Part model, mm, in its own coordinate system. A direction names the side the tool comes from. Give positions to 0.01 mm unless a question says otherwise; leave off trailing zeros. Write each loop counter-clockwise with the first axis right and the second up, starting at its lowest first coordinate (ties: lowest second). Pieces come first, ordered by that corner, then holes. Notation, with made-up numbers: M 16.5,8 L 40.5,8 A24 cw 40.5,33 Z; hole C 76,73.5 d6. An arc over 180 degrees is marked long. Use a Markdown table: item, result.
```python
from build123d import *

# Parameters (mm, degrees)
SKETCH_2_R          = 2.75
CUT_EXTRUDE_1_DEPTH = 10


with BuildPart() as part:
    # 草图1 → 旋转1 (revolve)
    with BuildSketch(Plane.XY, mode=Mode.PRIVATE) as revolve_1_sk:
        Polygon((-10, 0), (-32, 0), (-32, 8), (-20, 8), (-20, 32), (-10, 32), align=None)
    revolve(revolve_1_sk.sketch.rotate(Axis((0, 79.352678571, 0), (0, -1, 0)), 270), axis=Axis((0, 79.352678571, 0), (0, -1, 0)))

    # 草图2 → 切除-拉伸1 (cut)
    with BuildSketch(Plane(origin=(0, 8, 0), x_dir=(1, 0, 0), z_dir=(0, 1, 0))):
        with Locations(Location((0, 26, 0), (0, 0, 270))):
            Circle(SKETCH_2_R)
        with Locations(Location((26, 0, 0), (0, 0, 270))):
            Circle(SKETCH_2_R)
        with Locations(Location((0, -26, 0), (0, 0, 270))):
            Circle(SKETCH_2_R)
        with Locations(Location((-26, 0, 0), (0, 0, 270))):
            Circle(SKETCH_2_R)
    extrude(amount=-CUT_EXTRUDE_1_DEPTH, mode=Mode.SUBTRACT)


solid = part.part
```
1. Drop flat-ended pins along their axis: P1, Ø8, axis at x = 23, z = -10, coming from the +Y side; P2, Ø4, axis at y = 9, z = 24.5, coming from the -X side; P3, Ø5, axis at x = -26, z = 0, coming from the -Y side; P4, Ø2, axis at y = 17, z = 0, coming from the +X side. Give the stop position or say it passes through.
Findings below:
| item | result |
|---|---|
| P1 | y = 8 |
| P2 | x = -22.49 |
| P3 | through |
| P4 | x = 20 |
2. Drill centre lines: L1, parallel to X at y = 4, z = 0; L2, parallel to Y at x = -26.5, z = 3; L3, parallel to X at y = 2.25, z = -26. Where is each one in solid material? Low to high.
Findings below:
| item | result |
|---|---|
| L1 | -32 to -28.75, -23.25 to -10, 10 to 23.25, 28.75 to 32 |
| L2 | 0 to 8 |
| L3 | -18.65 to -2.75, 2.75 to 18.65 |
3. Tool access for faces 5 (the flat face through (-15, 8, 14)), 6 (the cylindrical face through (28.727, 4.056, -0.358)): list every direction of +Z, -Z, +X, -X, +Y, -Y with a clear straight run to the whole face (end or side of a thin tool).
Findings below:
| item | result |
|---|---|
| face 5 | +Y |
| face 6 | +Y, -Y |
4. Cut at B-B, the plane x = 0. Give the cut face in (y, z), then the cut area to 3 significant figures.
Findings below:
| item | result |
|---|---|
| outline | M 0,-32 L 8,-32 L 8,-28.75 L 0,-28.75 Z; M 0,-23.25 L 8,-23.25 L 8,-20 L 32,-20 L 32,-10 L 0,-10 Z; M 0,10 L 32,10 L 32,20 L 8,20 L 8,23.25 L 0,23.25 Z; M 0,28.75 L 8,28.75 L 8,32 L 0,32 Z |
| area | 744 mm2 |
5. Cut at C-C, the plane z = 26. Give the cut face in (x, y), then the cut area to 3 significant figures.
Findings below:
| item | result |
|---|---|
| outline | M -18.65,0 L -2.75,0 L -2.75,8 L -18.65,8 Z; M 2.75,0 L 18.65,0 L 18.65,8 L 2.75,8 Z |
| area | 254 mm2 |
6. Cut at A-A, the plane z = 0. Give the cut face in (x, y).
Findings below:
| item | result |
|---|---|
| outline | M -32,0 L -28.75,0 L -28.75,8 L -32,8 Z; M -23.25,0 L -10,0 L -10,32 L -20,32 L -20,8 L -23.25,8 Z; M 10,0 L 23.25,0 L 23.25,8 L 20,8 L 20,32 L 10,32 Z; M 28.75,0 L 32,0 L 32,8 L 28.75,8 Z |
7. Two-plate mould, pull along X, no slides. Class faces 1 (the cylindrical face through (-23.273, 4.056, -0.358)), 2 (the cylindrical face through (0.121, 4.056, 23.253)), 3 (the flat face through (-8, 0, -7)), 4 (the cylindrical face through (19.524, 20.168, -4.336)): released by +X, released by -X, zero draft, split by the parting line, or undercut.
Findings below:
| item | result |
|---|---|
| face 1 | undercut |
| face 2 | undercut |
| face 3 | zero draft |
| face 4 | split by the parting line |
8. Cut at D-D, the plane y = 4.5. Give the cut face in (x, z).
Findings below:
| item | result |
|---|---|
| outline | C 0,0 d64; hole C -26,0 d5.5; hole C 0,0 d20; hole C 0,-26 d5.5; hole C 0,26 d5.5; hole C 26,0 d5.5 |
